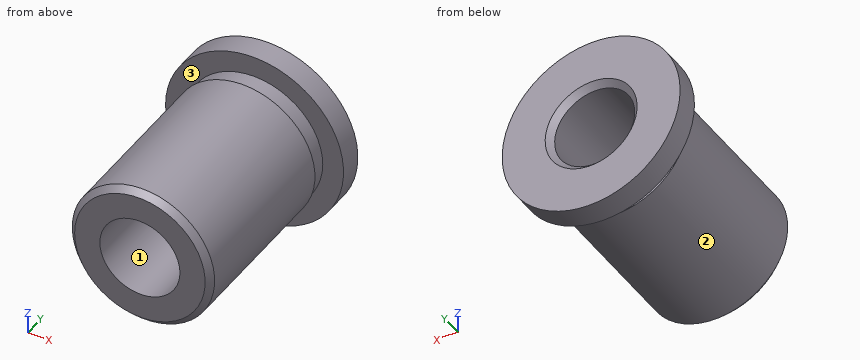
Autodesk Inventor part; units mm, degrees
ref_plane "YZ Plane" through (0, 0, 0) normal (1, 0, 0) x (0, 1, 0)
ref_plane "XZ Plane" through (0, 0, 0) normal (0, 1, 0) x (-1, 0, 0)
ref_plane "XY Plane" through (0, 0, 0) normal (0, 0, 1) x (1, 0, 0)
sketch "Sketch1" plane through (0, 0, 0) normal (0, 0, 1) x (1, 0, 0)
  line L0 (0, 0) -> (0, 18)
  line L1 (0, 0) -> (-6, 0)
  line L2 (-6, 0) -> (-6, 16)
  line L3 (-6, 16) -> (-7.5, 16)
  line L4 (-7.5, 16) -> (-7.5, 18)
  line L5 (-7.5, 18) -> (0, 18)
  dimension "d0" = 18
  dimension "d1" = 15
  dimension "d2" = 12
  dimension "d3" = 2
revolve "Revolution1" add sketch "Sketch1" angle 360 about axis through (0, 0, 0) along (0, 1, 0)
sketch "Sketch2" plane through (0, 0, 0) normal (0, 0, 1) x (1, 0, 0)
  line L0 (7.5, 16) -> (-7.5, 16)
  line L1 (-6, 0) -> (-6, 16)
  line L2 (-6, 14.5) -> (-5.75, 14.5)
  line L3 (-5.75, 14.5) -> (-5.75, 16)
  line L4 (0, 16) -> (0, 9.2067)
  point P0 (0, 0)
  dimension "d5" = 11.5
  dimension "d6" = 1.5
revolve "Revolution2" cut sketch "Sketch2" angle 360 about axis through (0, 16, 0) along (0, -1, 0)
sketch "Sketch3" plane through (0, 18, 0) normal (0, 1, 0) x (1, 0, 0)
  circle A0 centre (0, 0) radius 7.5
hole "d6.75" at (0, 18, 0) direction (0, -1, 0) diameter 6.75 end through all
chamfer "0.5x45" distance 0.5 angle 45 2 edges at (0, 18, -3.375) (6, 0, 0)
properties part number "s14-13" material "Steel, Carbon"
Read the model definition and answer for the solid it produces. Units are mm, in the model's axes. Face numbers are marked on the shaded views. Round coordinates to 2 decimals unless told otherwise and drop trailing zeros. Write each loop counter-clockwise with the first axis right and the second up, starting at its lowest first coordinate (ties: lowest second). Pieces come first, ordered by that corner, then holes. Notation, with made-up numbers: (52.5, -4) - (109.5, -4) arc R25 cw to (109.5, 31) - close; hole circle Ø7 at (-14, 21). An arc over 180 degrees is marked (long way). Use CSV: the item, a comma, the result in double quotes.
Q1. Find section A-A, the plane z = 0. Write down the section's boundary in (x, y) (3 decimals), then the cut area to 4 significant figures.
Values:
outline,"(-7.5, 16) - (-5.75, 16) - (-5.75, 14.5) - (-6, 14.5) - (-6, 0.5) - (-5.5, 0) - (-3.375, 0) - (-3.375, 17.5) - (-3.875, 18) - (-7.5, 18) - close; (3.375, 0) - (5.5, 0) - (6, 0.5) - (6, 14.5) - (5.75, 14.5) - (5.75, 16) - (7.5, 16) - (7.5, 18) - (3.875, 18) - (3.375, 17.5) - close"
area,"99.25 mm²"
Q2. Straight lines are drawn through the part: line 1 along Z through (x, y) = (0, 9.25) (3 decimals); line 2 along X through (y, z) = (11, -2.25). For each, find the intervals that lie inside material, in ascending order.
Values:
line 1,"z = -6 to -3.375, 3.375 to 6"
line 2,"x = -5.56 to -2.52, 2.52 to 5.56"
Q3. Find section B-B, the plane x = 0. Write down the section's boundary in (y, z) (3 decimals), then the cut area to 4 significant figures.
Values:
outline,"(0, -5.5) - (0.5, -6) - (14.5, -6) - (14.5, -5.75) - (16, -5.75) - (16, -7.5) - (18, -7.5) - (18, -3.875) - (17.5, -3.375) - (0, -3.375) - close; (0, 3.375) - (17.5, 3.375) - (18, 3.875) - (18, 7.5) - (16, 7.5) - (16, 5.75) - (14.5, 5.75) - (14.5, 6) - (0.5, 6) - (0, 5.5) - close"
area,"99.25 mm²"
Q4. Find section C-C, the plane y = 8.5. Write down the section's boundary in (x, z) (3 decimals).
Values:
outline,"circle Ø12 at (0, 0); hole circle Ø6.75 at (0, 0)"
Q5. Find section D-D, the plane x = -6.5. Write down the section's boundary in (y, z).
Values:
outline,"(16, -3.74) - (18, -3.74) - (18, 3.74) - (16, 3.74) - close"
Q6. Each of these flat-tipped pins is pushed along its axis until it touches: pin 1 Ø2 at (y, z) = (3.5, -6) entering from -X; pin 2 Ø6 at (x, y) = (2, 6) entering from -Z; pin 3 Ø4 at (y, z) = (13, 5.5) entering from -X. Where does it stop, or does it pass through?
Values:
pin 1,"stops at x = -3.32"
pin 2,"stops at z = -6"
pin 3,"stops at x = -4.87"
Q7. Determine the mould class of the marked faces 1, 2 and 3 for opening direction Z: +Z half, -Z half, draft (parallel to the pull), parting line (faces both ways), or undercut.
Values:
face 1,"undercut"
face 2,"parting line"
face 3,"draft"
